The listing builds one solid part. Answer for the finished solid, in the listing's coordinates (mm). A direction names the side the tool comes from. Coordinates: 2 decimals unless noted, no trailing zeros. Order: outer loops, then holes, each group sorted by start corner. A loop starts at its lowest first (then second) coordinate and runs counter-clockwise, first axis right, second up. Notation, with made-up numbers: (85.25, 53) -> (100.25, 53) arc R23 ccw to (100.25, 67) -> close; hole circle Ø4 at (-8.75, 18). An arc over 180 degrees is marked (long way). Answer in a Markdown table with one row per item.
```python
from build123d import *

# Parameters (mm, degrees)
SKETCH1_W           = 85
SKETCH1_H           = 20
SKETCH1_R           = 1.8
BOSS_EXTRUDE1_DEPTH = 7.4
CUT_EXTRUDE1_DEPTH  = 4.4
FILLET1_R           = 5


with BuildPart() as part:
    # Sketch1 → Boss-Extrude1 (new body)
    with BuildSketch(Plane.XY):
        Rectangle(SKETCH1_W, SKETCH1_H)
        with Locations((-32.5, 0)):
            Circle(SKETCH1_R, mode=Mode.SUBTRACT)
        with Locations((-22.5, 0)):
            Circle(SKETCH1_R, mode=Mode.SUBTRACT)
        with Locations((32.5, 0)):
            Circle(SKETCH1_R, mode=Mode.SUBTRACT)
        with Locations((22.5, 0)):
            Circle(SKETCH1_R, mode=Mode.SUBTRACT)
    extrude(amount=BOSS_EXTRUDE1_DEPTH)

    # Sketch2 → Cut-Extrude1 (cut)
    with BuildSketch(Plane(origin=(0, 0, 0), x_dir=(-1, 0, 0), z_dir=(0, 0, -1))):
        Polygon((20.652479139, -3.2), (18.804958277, 0), (20.652479139, 3.2), (24.347520861, 3.2), (26.195041723, 0), (24.347520861, -3.2), align=None)
        Polygon((36.195041723, 0), (34.347520861, 3.2), (30.652479139, 3.2), (28.804958277, 0), (30.652479139, -3.2), (34.347520861, -3.2), align=None)
        Polygon((-18.804958277, 0), (-20.652479139, 3.2), (-24.347520861, 3.2), (-26.195041723, 0), (-24.347520861, -3.2), (-20.652479139, -3.2), align=None)
        Polygon((-34.347520861, -3.2), (-36.195041723, 0), (-34.347520861, 3.2), (-30.652479139, 3.2), (-28.804958277, 0), (-30.652479139, -3.2), align=None)
    extrude(amount=-CUT_EXTRUDE1_DEPTH, mode=Mode.SUBTRACT)

    # Fillet1
    fillet1_edges = [part.edges().sort_by_distance(p)[0] for p in [
        (0, -10, 0),
    ]]
    fillet(fillet1_edges, radius=FILLET1_R)


solid = part.part
```
(1) A cutting plane is placed at D-D, the plane z = 2. Determine the outline of the cut face in (x, y), then the cut area to 3 significant figures.
Check values:
| item | result |
|---|---|
| outline | (-42.5, -9) -> (42.5, -9) -> (42.5, 10) -> (-42.5, 10) -> close; hole (-36.2, 0) -> (-34.35, -3.2) -> (-30.65, -3.2) -> (-28.8, 0) -> (-30.65, 3.2) -> (-34.35, 3.2) -> close; hole (-26.2, 0) -> (-24.35, -3.2) -> (-20.65, -3.2) -> (-18.8, 0) -> (-20.65, 3.2) -> (-24.35, 3.2) -> close; hole (18.8, 0) -> (20.65, -3.2) -> (24.35, -3.2) -> (26.2, 0) -> (24.35, 3.2) -> (20.65, 3.2) -> close; hole (28.8, 0) -> (30.65, -3.2) -> (34.35, -3.2) -> (36.2, 0) -> (34.35, 3.2) -> (30.65, 3.2) -> close |
| area | 1,470 mm² |
(2) A cutting plane is placed at C-C, the plane x = -12.5. Determine the outline of the cut face in (y, z), then the cut area to 3 significant figures.
Check values:
| item | result |
|---|---|
| outline | (-10, 5) arc R5 ccw to (-5, 0) -> (10, 0) -> (10, 7.4) -> (-10, 7.4) -> close |
| area | 143 mm² |
(3) Flat-ended cylindrical pins translate along their axes: pin 1 (3 mm diameter, centred on x = 32, y = -1, fed in from -Z); pin 2 (1.8 mm diameter, centred on x = -22.5, z = 1, fed in from -Y); pin 3 (1.8 mm diameter, centred on x = 22.5, z = 2, fed in from -Y); pin 4 (2 mm diameter, centred on x = -32.5, y = 0, fed in from +Z). Find the tip coordinate at first contact, or state that the pin passes through.
Check values:
| item | result |
|---|---|
| pin 1 | z = 4.4 |
| pin 2 | y = -8.92 |
| pin 3 | y = -9.54 |
| pin 4 | through |
(4) A cutting plane is placed at A-A, the plane z = 6.25. Determine the outline of the cut face in (x, y), then the cut area to 3 significant figures.
Check values:
| item | result |
|---|---|
| outline | (-42.5, -10) -> (42.5, -10) -> (42.5, 10) -> (-42.5, 10) -> close; hole circle Ø3.6 at (-32.5, 0); hole circle Ø3.6 at (-22.5, 0); hole circle Ø3.6 at (22.5, 0); hole circle Ø3.6 at (32.5, 0) |
| area | 1,660 mm² |
(5) Find the intervals of material crossed by line 1 along X through (y, z) = (0, 6); line 2 along Y through (x, z) = (-32.5, 6.35); line 3 along X through (y, z) = (-1.75, 0.75), in increasing order. Write a range as from..to.
Check values:
| item | result |
|---|---|
| line 1 | -42.5..-34.3, -30.7..-24.3, -20.7..20.7, 24.3..30.7, 34.3..42.5 |
| line 2 | -10..-1.8, 1.8..10 |
| line 3 | -42.5..-35.18, -29.82..-25.18, -19.82..19.82, 25.18..29.82, 35.18..42.5 |
(6) Which of the six approach directions +Z, -Z, +X, -X, +Y, -Y give full straight-line access (tool end or side, diameter ignored) to faces 1 (the flat face through (32, -3.2, 2)), 2 (the cylindrical face through (-30.783, 0.541, 5.879))?
Check values:
| item | result |
|---|---|
| face 1 | -Z |
| face 2 | +Z, -Z |
(7) For a pull along Y with two mould halves and no side action, classify faces 3 (the cylindrical face through (1, -9, 2)), 4 (the flat face through (-33, 3.2, 2)), 5 (the flat face through (-1, 0, 7.4)) as released by +Y, released by -Y, zero draft, split by the parting line, or undercut.
Check values:
| item | result |
|---|---|
| face 3 | released by -Y |
| face 4 | undercut |
| face 5 | zero draft |
(8) A cutting plane is placed at B-B, the plane x = -32.5. Determine the outline of the cut face in (y, z), then the cut area to 3 significant figures.
Check values:
| item | result |
|---|---|
| outline | (-10, 5) arc R5 ccw to (-5, 0) -> (-3.2, 0) -> (-3.2, 4.4) -> (-1.8, 4.4) -> (-1.8, 7.4) -> (-10, 7.4) -> close; (1.8, 4.4) -> (3.2, 4.4) -> (3.2, 0) -> (10, 0) -> (10, 7.4) -> (1.8, 7.4) -> close |
| area | 104 mm² |
